```python
from build123d import *

# Parameters (mm, degrees)
BOSS_EXTRUDE1_DEPTH = 7.8
FILLET1_R           = 1
SKETCH3_R           = 2.4
BOSS_EXTRUDE2_DEPTH = 5.5
SHELL3_START        = 1.25
SHELL3_DEPTH        = 5.3
SHELL3_START_2      = 12.45
SHELL3_2_OUTLINE_R  = 1.15
SHELL3_2_DEPTH      = 5.5
SKETCH7_R           = 1.9
CUT_EXTRUDE5_DEPTH  = 2
BOSS_EXTRUDE3_REACH = 24.091


with BuildPart() as part:
    # Sketch2 → Boss-Extrude1 (new body)
    with BuildSketch(Plane.XY):
        Polygon((-7.65, 0), (7.65, 0), (7.65, 1), (5.599872407, 13.7), (2.399872407, 13.7), (-2.399872407, 13.7), (-5.599872407, 13.7), (-7.65, 1), align=None)
    extrude(amount=BOSS_EXTRUDE1_DEPTH)

    # Fillet1
    fillet1_edges = [part.edges().sort_by_distance(p)[0] for p in [
        (5.599872407, 13.7, 3.9),
        (0, 13.7, 7.8),
        (-5.599872407, 13.7, 3.9),
        (0, 13.7, 0),
        (6.624936203, 7.35, 0),
        (6.624936203, 7.35, 7.8),
        (-6.624936203, 7.35, 7.8),
        (-6.624936203, 7.35, 0),
    ]]
    fillet(fillet1_edges, radius=FILLET1_R)

    # Sketch3 → Boss-Extrude2 (add)
    with BuildSketch(Plane(origin=(0, 13.7, 0), x_dir=(1, 0, 0), z_dir=(0, 1, 0))):
        with Locations((0, -3.9)):
            Circle(SKETCH3_R)
    extrude(amount=BOSS_EXTRUDE2_DEPTH)

    # Shell3: read off the stored shape, not the designer's step
    # Shell3 outline → Shell3 (cut)
    with BuildSketch(Plane.XY.offset(SHELL3_START)):
        Polygon((6.4, 0), (6.4, 0.899756749), (4.535474615, 12.45), (-4.535474615, 12.45), (-6.4, 0.899756749), (-6.4, 0), align=None)
    extrude(amount=SHELL3_DEPTH, mode=Mode.SUBTRACT)

    # Shell3 2 outline → Shell3 2 (cut)
    with BuildSketch(Plane(origin=(0, 0, 0), x_dir=(1, 0, 0), z_dir=(0, 1, 0)).offset(SHELL3_START_2)):
        with Locations((0, -3.9)):
            Circle(SHELL3_2_OUTLINE_R)
    extrude(amount=SHELL3_2_DEPTH, mode=Mode.SUBTRACT)

    # Sketch7 → Cut-Extrude5 (cut)
    with BuildSketch(Plane(origin=(7.613040698, 1.228953134, 0), x_dir=(0, 0, -1), z_dir=(0.987219843348776, 0.15936430245954794, 0))):
        with Locations(Location((-4, 7.98097386, 0), (0, 0, 90))):
            Circle(SKETCH7_R)
    cut_extrude5 = extrude(amount=-CUT_EXTRUDE5_DEPTH, mode=Mode.SUBTRACT)

    # Mirror1: Cut-Extrude5 across plane
    add(cut_extrude5.mirror(Plane(origin=(0, 0, 0), x_dir=(0, 0, 1), z_dir=(1, 0, 0))), mode=Mode.SUBTRACT)

    # Sketch8 → Boss-Extrude3 (add, up to next)
    with BuildSketch(Plane.XZ, mode=Mode.PRIVATE) as boss_extrude3_sk1:
        with BuildLine():
            Line((1.5, 6.55), (1.5, 5.692944235))
            ThreePointArc((1.5, 5.692944235), (2.274557316, 5.926727718), (2.790430764, 6.55))
            Line((2.790430764, 6.55), (1.5, 6.55))
        make_face()
    boss_extrude3_tool1 = extrude(boss_extrude3_sk1.sketch, amount=-BOSS_EXTRUDE3_REACH, mode=Mode.PRIVATE) - part.part
    # Sketch8 → Boss-Extrude3 (add, up to next)
    with BuildSketch(Plane.XZ, mode=Mode.PRIVATE) as boss_extrude3_sk2:
        with BuildLine():
            Line((-1.5, 6.55), (-1.5, 5.692944235))
            ThreePointArc((-1.5, 5.692944235), (-2.274557316, 5.926727718), (-2.790430764, 6.55))
            Line((-2.790430764, 6.55), (-1.5, 6.55))
        make_face()
    boss_extrude3_tool2 = extrude(boss_extrude3_sk2.sketch, amount=-BOSS_EXTRUDE3_REACH, mode=Mode.PRIVATE) - part.part
    # Sketch8 → Boss-Extrude3 (add, up to next)
    with BuildSketch(Plane.XZ, mode=Mode.PRIVATE) as boss_extrude3_sk3:
        with BuildLine():
            Line((1.5, 1.25), (1.5, 2.107055765))
            ThreePointArc((1.5, 2.107055765), (2.274557316, 1.873272282), (2.790430764, 1.25))
            Line((2.790430764, 1.25), (1.5, 1.25))
        make_face()
    boss_extrude3_tool3 = extrude(boss_extrude3_sk3.sketch, amount=-BOSS_EXTRUDE3_REACH, mode=Mode.PRIVATE) - part.part
    # Sketch8 → Boss-Extrude3 (add, up to next)
    with BuildSketch(Plane.XZ, mode=Mode.PRIVATE) as boss_extrude3_sk4:
        with BuildLine():
            Line((-1.5, 1.25), (-1.5, 2.107055765))
            ThreePointArc((-1.5, 2.107055765), (-2.274557316, 1.873272282), (-2.790430764, 1.25))
            Line((-2.790430764, 1.25), (-1.5, 1.25))
        make_face()
    boss_extrude3_tool4 = extrude(boss_extrude3_sk4.sketch, amount=-BOSS_EXTRUDE3_REACH, mode=Mode.PRIVATE) - part.part
    add(boss_extrude3_tool1.solids().sort_by_distance((2.012361, 0, 6.196212))[0])
    add(boss_extrude3_tool2.solids().sort_by_distance((-2.012361, 0, 6.196212))[0])
    add(boss_extrude3_tool3.solids().sort_by_distance((2.012361, 0, 1.603788))[0])
    add(boss_extrude3_tool4.solids().sort_by_distance((-2.012361, 0, 1.603788))[0])


solid = part.part
```
Part model, mm, in its own coordinate system. A direction names the side the tool comes from. Coordinates: 2 decimals unless noted, no trailing zeros. Write each loop counter-clockwise with the first axis right and the second up, starting at its lowest first coordinate (ties: lowest second). Pieces come first, ordered by that corner, then holes.
Item 1: Mould opens along X. For faces 1 (the face through (-5.389, 13.468, 3.941)), 2 (the face through (5.404, 13.455, 3.941)), 3 (the face through (5.48, 6.59, 3.86)) say: released by +X, released by -X, zero draft, split by the parting line, or undercut.
Item 2: Pin check, flat tips, straight feed: pin 1 (0.7 mm diameter, centred on y = 7, z = 2, fed in from -X); pin 2 (2.5 mm diameter, centred on x = -0.5, z = 4.5, fed in from -Y); pin 3 (1.5 mm diameter, centred on y = 17, z = 3, fed in from +X). Stop position of each tip, or through.
Item 3: Slice it at C-C (y = 17). Write the cut outline in (x, z), and give its area (3 significant figures).
Item 4: Which spindle directions (+Z, -Z, +X, -X, +Y, -Y) get a long thin tool onto all of the face, cutting with end or side? Do faces 4 (the face through (-1.5, 6, 6)), 5 (the face through (-5.57, 10.02, 5.6)). Say none if no direction does.
Item 5: Probe line 1 (X direction, y = 16.75, z = 4); line 2 (Z direction, x = 0, y = 14.35); line 3 (Z direction, x = -4, y = 2). List the from-to ranges inside material, lowest first.
Item 6: Slice it at B-B (x = 0). Write the cut outline in (y, z).
Item 7: Slice it at D-D (z = 4.25). Count the separate pieces of the cut face and the enclosed holes in it, and give its area (3 significant figures).
Item 8: Slice it at A-A (z = 2.5). Write the cut outline in (x, y), and give its area (3 significant figures).
Results found:
1. face 1: released by -X
1. face 2: released by +X
1. face 3: undercut
2. pin 1: stops at x = -6.74
2. pin 2: stops at y = 12.45
2. pin 3: stops at x = 2.4
3. outline: circle Ø4.8 at (0, 3.9); hole circle Ø2.3 at (0, 3.9)
3. area: 13.9 mm2
4. face 4: -Y
4. face 5: none
5. line 1: x = -2.4 to -1.15, 1.15 to 2.4
5. line 2: z = 1.5 to 2.75, 5.05 to 6.3
5. line 3: z = 0 to 1.25, 6.55 to 7.8
6. outline: (0, 0) - (12.7, 0) arc R1 ccw to (13.7, 1) - (13.7, 1.5) - (19.2, 1.5) - (19.2, 6.3) - (13.7, 6.3) - (13.7, 6.8) arc R1 ccw to (12.7, 7.8) - (0, 7.8) - (0, 6.55) - (12.45, 6.55) - (12.45, 5.05) - (17.95, 5.05) - (17.95, 2.75) - (12.45, 2.75) - (12.45, 1.25) - (0, 1.25) - close
7. separate pieces: 3
7. enclosed holes: 0
7. area: 50.1 mm2
8. outline: (-7.65, 0) - (-6.4, 0) - (-6.4, 0.9) - (-5.29, 7.76) - (-6.53, 7.96) - (-7.65, 1) - close; (-6.16, 10.26) - (-4.92, 10.06) - (-4.54, 12.45) - (4.54, 12.45) - (4.92, 10.06) - (6.16, 10.26) - (5.74, 12.86) arc R1 ccw to (4.75, 13.7) - (1.95, 13.7) - (1.95, 19.2) - (-1.95, 19.2) - (-1.95, 13.7) - (-4.75, 13.7) arc R1 ccw to (-5.74, 12.86) - close; (5.29, 7.76) - (6.4, 0.9) - (6.4, 0) - (7.65, 0) - (7.65, 1) - (6.53, 7.96) - close
8. area: 61.1 mm2
